Build history of the part. All positions in model axes, mm. A direction names the side the tool comes from. Give positions to 0.01 mm unless a question says otherwise; leave off trailing zeros. Write each loop counter-clockwise with the first axis right and the second up, starting at its lowest first coordinate (ties: lowest second). Pieces come first, ordered by that corner, then holes. Notation, with made-up numbers: M -9,-23 L 40,-23 A15 ccw 40,-8 Z; hole C 73,39 d3. An arc over 180 degrees is marked long. Return JSON: item names as keys, results as strings. Group by question number.
Q1. Band-saw the part on B-B, the plane z = 76.2. Give the cut face in (x, y), then the cut area to 3 significant figures.
Q2. Band-saw the part on A-A, the plane x = 7.25. Count the separate pieces of the cut face and the enclosed holes in it, then the cut area to 3 significant figures.
Q3. Tool access for faces 1 (the flat face through (6, -6.35, -2)), 2 (the cylindrical face through (-9.57, 14.24, 119.64)), 3 (the cylindrical face through (3.042, 19.876, 22.332)): list every direction of +Z, -Z, +X, -X, +Y, -Y with a clear straight run to the whole face (end or side of a thin tool).
Q4. Band-saw the part on C-C, the plane z = -12.7. Give the cut face in (x, y) (3 decimals), then the cut area to 3 significant figures.
Q5. Pull direction Y, two halves, no side cores. Call faces 4 (the flat face through (0, -25.4, -2)), 5 (the flat face through (12.7, -16, 2)), 6 (the cylindrical face through (-2.5, 0.69, 15.8)): +Y half, -Y half, draft (parallel to the pull), parting line (faces both ways), or undercut.
Q6. Wall check: probe 1 along Y at (x, z) = (10, -9); probe 2 along Y at (x, z) = (-2.8, 12.7) (3 decimals); probe 3 along X at (y, z) = (-0.5, 9.5). Give the ranges that are in metal, low to high.
Q7. Flat gauge pins, fed straight in: pin 1 Ø9 at (y, z) = (0, -88.9) entering from +X; pin 2 Ø7.5 at (y, z) = (-19, -77) entering from -X; pin 3 Ø4.5 at (y, z) = (16.5, 23) entering from -X. Where does each tip first touch, or does it go through?
from build123d import *

# Parameters (mm, degrees)
F0_W      = 50.8
F0_H      = 304.8
F1_DEPTH  = 12.7
F3_W      = 12.7
F3_H      = 12.7
F4_DEPTH  = 304.8
F7_D      = 10.0838
F7_DEPTH  = 30.48
F7_TIP    = 3.0294791551
F9_R      = 7.54126
F9_R_2    = 3.302
F10_DEPTH = 6.35
F12_D     = 6.35
F12_DEPTH = 30.48
F12_TIP   = 1.9077324654
F13_R     = 5.0419
F13_R_2   = 2.54
F14_DEPTH = 7.62


# Not quite as in the source:
# - a feature names something its author has since deleted; it is built from what else it names


with BuildPart() as f1:
    # F0 (on Right) → F1 (new body, symmetric)
    with BuildSketch(Plane.YZ):
        Rectangle(F0_W, F0_H)
    extrude(amount=F1_DEPTH, both=True)

    # F3 (on offset) → F4 (cut)
    with BuildSketch(Plane.XY.offset(-152.4)):
        with Locations((6.35, 0)):
            Rectangle(F3_W, F3_H)
    extrude(amount=F4_DEPTH, mode=Mode.SUBTRACT)

    # F7
    with Locations(Plane.YZ.offset(12.7)):
        with Locations((-15.875, 76.2), (15.875, 76.2), (15.875, 25.4), (-15.875, 25.4), (-15.875, -25.4), (15.875, -25.4), (15.875, -127), (-15.875, -127), (-15.875, -76.2), (15.875, -76.2), (-15.875, 127), (15.875, 127)):
            Hole(F7_D / 2, depth=F7_DEPTH)
            with Locations((0, 0, -(F7_DEPTH + F7_TIP / 2))):  # 118° drill point
                Cone(0, F7_D / 2, F7_TIP, mode=Mode.SUBTRACT)

    # F9 (on offset) → F10 (cut)
    with BuildSketch(Plane.YZ.offset(-12.7)):
        with Locations((15.875, 127)):
            Circle(F9_R)
        with Locations((15.875, 127)):
            Circle(F9_R_2, mode=Mode.SUBTRACT)
        with Locations((-15.875, 127)):
            Circle(F9_R)
        with Locations((-15.875, 127)):
            Circle(F9_R_2, mode=Mode.SUBTRACT)
        with Locations((-15.875, 76.2)):
            Circle(F9_R)
        with Locations((-15.875, 76.2)):
            Circle(F9_R_2, mode=Mode.SUBTRACT)
        with Locations((15.875, 76.2)):
            Circle(F9_R)
        with Locations((15.875, 76.2)):
            Circle(F9_R_2, mode=Mode.SUBTRACT)
        with Locations((15.875, 25.4)):
            Circle(F9_R)
        with Locations((15.875, 25.4)):
            Circle(F9_R_2, mode=Mode.SUBTRACT)
        with Locations((-15.875, 25.4)):
            Circle(F9_R)
        with Locations((-15.875, 25.4)):
            Circle(F9_R_2, mode=Mode.SUBTRACT)
        with Locations((15.875, -25.4)):
            Circle(F9_R)
        with Locations((15.875, -25.4)):
            Circle(F9_R_2, mode=Mode.SUBTRACT)
        with Locations((-15.875, -25.4)):
            Circle(F9_R)
        with Locations((-15.875, -25.4)):
            Circle(F9_R_2, mode=Mode.SUBTRACT)
        with Locations((-15.875, -76.2)):
            Circle(F9_R)
        with Locations((-15.875, -76.2)):
            Circle(F9_R_2, mode=Mode.SUBTRACT)
        with Locations((15.875, -76.2)):
            Circle(F9_R)
        with Locations((15.875, -76.2)):
            Circle(F9_R_2, mode=Mode.SUBTRACT)
        with Locations((15.875, -127)):
            Circle(F9_R)
        with Locations((15.875, -127)):
            Circle(F9_R_2, mode=Mode.SUBTRACT)
        with Locations((-15.875, -127)):
            Circle(F9_R)
        with Locations((-15.875, -127)):
            Circle(F9_R_2, mode=Mode.SUBTRACT)
    extrude(amount=F10_DEPTH, mode=Mode.SUBTRACT)

    # F12
    with Locations(Plane(origin=(-12.7, 0, 0), x_dir=(0, 1, 0), z_dir=(-1, 0, 0))):
        with Locations((0, -139.7), (0, -114.3), (0, -88.9), (0, -63.5), (0, -38.1), (0, 12.7), (0, -12.7), (0, 38.1), (0, 63.5), (0, 114.3), (0, 139.7), (0, 88.9)):
            Hole(F12_D / 2, depth=F12_DEPTH)
            with Locations((0, 0, -(F12_DEPTH + F12_TIP / 2))):  # 118° drill point
                Cone(0, F12_D / 2, F12_TIP, mode=Mode.SUBTRACT)

    # F13 (on offset) → F14 (cut)
    with BuildSketch(Plane.YZ.offset(-12.7)):
        with Locations((0, 139.7)):
            Circle(F13_R)
        with Locations((0, 139.7)):
            Circle(F13_R_2, mode=Mode.SUBTRACT)
        with Locations((0, 114.3)):
            Circle(F13_R)
        with Locations((0, 114.3)):
            Circle(F13_R_2, mode=Mode.SUBTRACT)
        with Locations((0, 88.9)):
            Circle(F13_R)
        with Locations((0, 88.9)):
            Circle(F13_R_2, mode=Mode.SUBTRACT)
        with Locations((0, 63.5)):
            Circle(F13_R)
        with Locations((0, 63.5)):
            Circle(F13_R_2, mode=Mode.SUBTRACT)
        with Locations((0, 38.1)):
            Circle(F13_R)
        with Locations((0, 38.1)):
            Circle(F13_R_2, mode=Mode.SUBTRACT)
        with Locations((0, 12.7)):
            Circle(F13_R)
        with Locations((0, 12.7)):
            Circle(F13_R_2, mode=Mode.SUBTRACT)
        with Locations((0, -12.7)):
            Circle(F13_R)
        with Locations((0, -12.7)):
            Circle(F13_R_2, mode=Mode.SUBTRACT)
        with Locations((0, -38.1)):
            Circle(F13_R)
        with Locations((0, -38.1)):
            Circle(F13_R_2, mode=Mode.SUBTRACT)
        with Locations((0, -63.5)):
            Circle(F13_R)
        with Locations((0, -63.5)):
            Circle(F13_R_2, mode=Mode.SUBTRACT)
        with Locations((0, -88.9)):
            Circle(F13_R)
        with Locations((0, -88.9)):
            Circle(F13_R_2, mode=Mode.SUBTRACT)
        with Locations((0, -114.3)):
            Circle(F13_R)
        with Locations((0, -114.3)):
            Circle(F13_R_2, mode=Mode.SUBTRACT)
        with Locations((0, -139.7)):
            Circle(F13_R)
        with Locations((0, -139.7)):
            Circle(F13_R_2, mode=Mode.SUBTRACT)
    extrude(amount=F14_DEPTH, mode=Mode.SUBTRACT)


solid = f1.part
From the geometry:
{
 "1": {"outline": "M -12.7,-25.4 L 12.7,-25.4 L 12.7,-20.92 L -6.35,-20.92 L -6.35,-23.42 L -12.7,-23.42 Z; M -12.7,-8.33 L -6.35,-8.33 L -6.35,-10.83 L 12.7,-10.83 L 12.7,-6.35 L 0,-6.35 L 0,6.35 L 12.7,6.35 L 12.7,10.83 L -6.35,10.83 L -6.35,8.33 L -12.7,8.33 Z; M -12.7,23.42 L -6.35,23.42 L -6.35,20.92 L 12.7,20.92 L 12.7,25.4 L -12.7,25.4 Z", "area": "553 mm^2"},
 "2": {"separate pieces": "2", "enclosed holes": "12", "area": "10,700 mm^2"},
 "3": {"face 1": "+Z, -Z, +X", "face 2": "-X", "face 3": "+X, -X"},
 "4": {"outline": "M -12.7,-25.4 L 12.7,-25.4 L 12.7,-6.35 L 0,-6.35 L 0,-3.175 L -5.08,-3.175 L -5.08,-5.042 L -12.7,-5.042 Z; M -12.7,5.042 L -5.08,5.042 L -5.08,3.175 L 0,3.175 L 0,6.35 L 12.7,6.35 L 12.7,25.4 L -12.7,25.4 Z", "area": "1,020 mm^2"},
 "5": {"face 4": "-Y half", "face 5": "draft", "face 6": "undercut"},
 "6": {"probe 1": "y = -25.4 to -6.35, 6.35 to 25.4", "probe 2": "y = -25.4 to -3.175, 3.175 to 25.4", "probe 3": "x = -5.08 to 0"},
 "7": {"pin 1": "stops at x = 0", "pin 2": "stops at x = -6.35", "pin 3": "passes through"}
}
